```python
from build123d import *

# Parameters (mm, degrees)
F0_W     = 120
F0_H     = 60
F1_DEPTH = 12
F2_R     = 10
F4_DEPTH = 10


with BuildPart() as f1:
    # F0 (on Top) → F1 (new body)
    with BuildSketch(Plane.XY):
        with Locations((7.758874, -6.406293)):
            Rectangle(F0_W, F0_H)
    extrude(amount=F1_DEPTH)

    # F2
    f2_edges = [f1.edges().sort_by_distance(p)[0] for p in [
        (-52.241126, -36.406293, 6),
        (67.758874, -36.406293, 6),
        (67.758874, 23.593707, 6),
        (-52.241126, 23.593707, 6),
    ]]
    fillet(f2_edges, radius=F2_R)

    # F3 (on face) → F4 (cut)
    with BuildSketch(Plane.XY.offset(12)):
        with BuildLine():
            Line((65.758874, -26.406293), (65.758874, 13.593707))
            ThreePointArc((65.758874, 13.593707), (63.415729, 19.250562), (57.758874, 21.593707))
            Line((57.758874, 21.593707), (-42.241126, 21.593707))
            ThreePointArc((-42.241126, 21.593707), (-47.89798, 19.250562), (-50.241126, 13.593707))
            Line((-50.241126, 13.593707), (-50.241126, -26.406293))
            ThreePointArc((-50.241126, -26.406293), (-47.89798, -32.063147), (-42.241126, -34.406293))
            Line((-42.241126, -34.406293), (57.758874, -34.406293))
            ThreePointArc((57.758874, -34.406293), (63.415729, -32.063147), (65.758874, -26.406293))
        make_face()
    extrude(amount=-F4_DEPTH, mode=Mode.SUBTRACT)


solid = f1.part
```
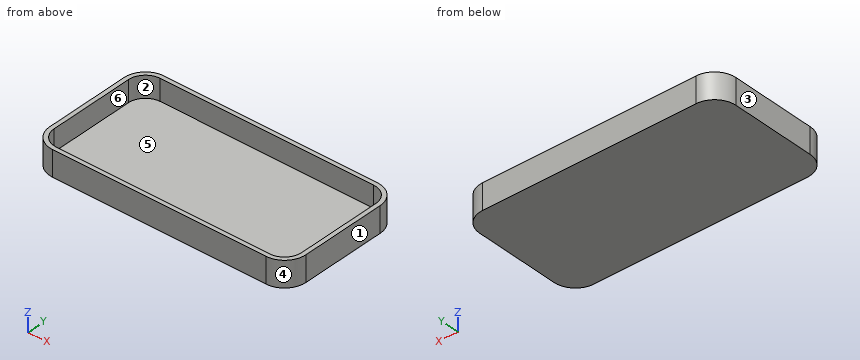
Can you work these out from the model? Positions are in its coordinate system, mm. Face numbers are marked on the shaded views. A direction names the side the tool comes from. Coordinates: 2 decimals unless noted, no trailing zeros. Loops run counter-clockwise (first coordinate to the right, second up) from the corner with the lowest first, then second, coordinate; pieces in that order, holes last.
Item 1: Suppose I cut it at A-A (z = 3.25). Please give me the cut outline in (x, y).
Answers below:
outline: (-52.24, -26.41) arc R10 ccw to (-42.24, -36.41) - (57.76, -36.41) arc R10 ccw to (67.76, -26.41) - (67.76, 13.59) arc R10 ccw to (57.76, 23.59) - (-42.24, 23.59) arc R10 ccw to (-52.24, 13.59) - close; hole (-50.24, -26.41) arc R8 ccw to (-42.24, -34.41) - (57.76, -34.41) arc R8 ccw to (65.76, -26.41) - (65.76, 13.59) arc R8 ccw to (57.76, 21.59) - (-42.24, 21.59) arc R8 ccw to (-50.24, 13.59) - close
Item 2: I'm going to push a flat-ended pin straight in: pin 1 (10 mm diameter, centred on x = 12, y = -7, fed in from +Z). Where does the tip first touch, or does it pass through?
Answers below:
pin 1: stops at z = 2
Item 3: Which directions (+Z, -Z, +X, -X, +Y, -Y) give clear straight access to the entire face, cutting with the end or side of a thin tool? Please do the marked faces 1 and 2.
Answers below:
face 1: +Z, -Z, +X, +Y, -Y
face 2: +Z
Item 4: Suppose I cut it at C-C (y = 2). Please give me the cut outline in (x, z), then the cut area to 3 significant figures.
Answers below:
outline: (-52.24, 0) - (67.76, 0) - (67.76, 12) - (65.76, 12) - (65.76, 2) - (-50.24, 2) - (-50.24, 12) - (-52.24, 12) - close
area: 280 mm2
Item 5: If we mould it in two halves opening along Y, with no side actions, what happens to the marked faces 3, 4, 5 and 6? For each: released by +Y, released by -Y, zero draft, split by the parting line, or undercut.
Answers below:
face 3: zero draft
face 4: released by -Y
face 5: undercut
face 6: undercut
Item 6: Suppose I cut it at B-B (x = 35). Please give me the cut outline in (y, z).
Answers below:
outline: (-36.41, 0) - (23.59, 0) - (23.59, 12) - (21.59, 12) - (21.59, 2) - (-34.41, 2) - (-34.41, 12) - (-36.41, 12) - close
Item 7: Please list where these lines run through material, in increasing order: L1, parallel to Y at x = 11.5, z = 9.5; L2, parallel to X at y = -22, z = 10; L3, parallel to Z at x = 22.5, y = 12.
Answers below:
L1: y = -36.41 to -34.41, 21.59 to 23.59
L2: x = -52.24 to -50.24, 65.76 to 67.76
L3: z = 0 to 2
